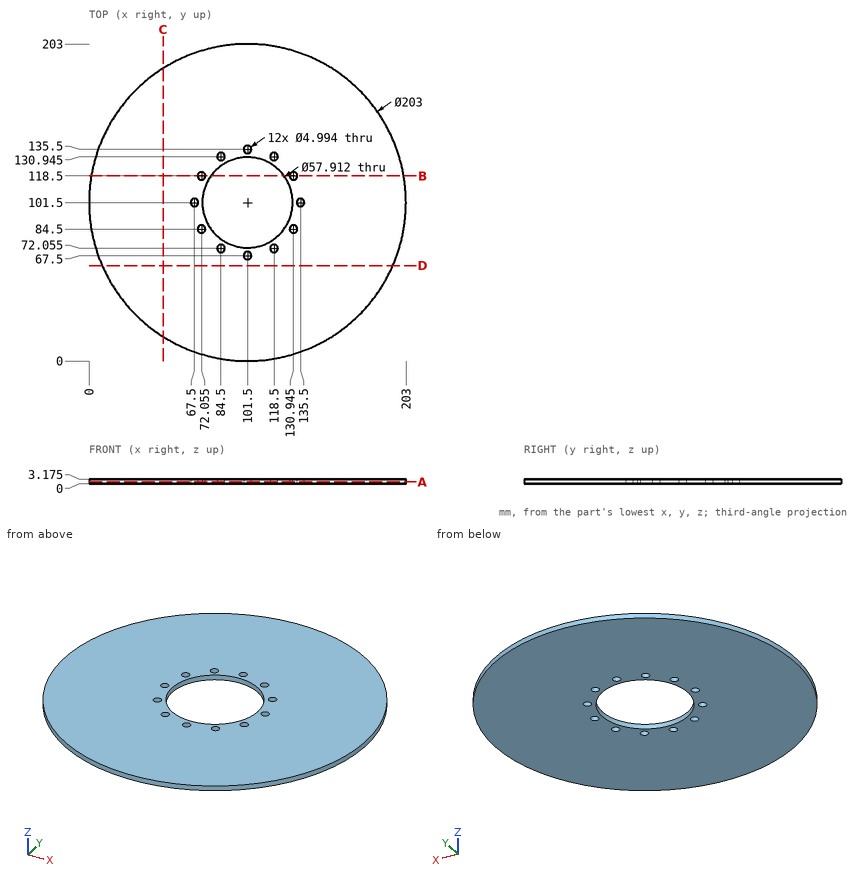
Answer from the drawing. Dimensions are ordinates in mm from the lowest x, y and z of the part. Coordinates: 2 decimals unless noted, no trailing zeros. Order: outer loops, then holes, each group sorted by start corner. A loop starts at its lowest first (then second) coordinate and runs counter-clockwise, first axis right, second up. Notation, with made-up numbers: (49.5, 38.25) -> (78.5, 38.25) arc R32 ccw to (78.5, 72.25) -> close; hole circle Ø9 at (5, -14.75). An arc over 180 degrees is marked (long way). Answer as a JSON object with one key per item and string values.
1) A cutting plane is placed at C-C, the plane x = 47.5. Determine the outline of the cut face in (y, z) (1 decimal), plus the area to 3 significant figures.
Model answer:
{"outline": "(15.6, 0) -> (187.4, 0) -> (187.4, 3.2) -> (15.6, 3.2) -> close", "area": "546 mm²"}
2) A cutting plane is placed at A-A, the plane z = 1.35. State how many separate pieces and enclosed holes the cut face has, plus the area to 3 significant figures.
Model answer:
{"separate pieces": "1", "enclosed holes": "13", "area": "29,500 mm²"}
3) Consider line 1 along X through (y, z) = (102, 2.3); line 2 along Y through (x, z) = (101.5, 2); line 3 along Y through (x, z) = (85.5, 2.3). Determine where each line is inside the solid, lowest interval first. Write a range as from..to.
Model answer:
{"line 1": "x = 0..65.05, 69.95..72.55, 130.45..133.05, 137.95..203", "line 2": "y = 0..65, 70..72.54, 130.46..133, 138..203", "line 3": "y = 1.27..69.77, 74.34..77.37, 125.63..128.66, 133.23..201.73"}
4) A cutting plane is placed at B-B, the plane y = 118.5. Determine the outline of the cut face in (x, z) (1 decimal), plus the area to 3 significant figures.
Model answer:
{"outline": "(1.4, 0) -> (69.6, 0) -> (69.6, 3.2) -> (1.4, 3.2) -> close; (74.6, 0) -> (78.1, 0) -> (78.1, 3.2) -> (74.6, 3.2) -> close; (124.9, 0) -> (128.4, 0) -> (128.4, 3.2) -> (124.9, 3.2) -> close; (133.4, 0) -> (201.6, 0) -> (201.6, 3.2) -> (133.4, 3.2) -> close", "area": "455 mm²"}
5) Each of these flat-tipped pins is pushed along its axis until it touches: pin 1 (4 mm diameter, centred on x = 67.5, y = 101.5, fed in from +Z); pin 2 (1.5 mm diameter, centred on x = 74.5, z = 1.5, fed in from -Y). Where does it stop, or does it pass through?
Model answer:
{"pin 1": "passes through", "pin 2": "stops at y = 3.45"}
6) A cutting plane is placed at D-D, the plane y = 61. Determine the outline of the cut face in (x, z) (3 decimals).
Model answer:
{"outline": "(8.43, 0) -> (194.57, 0) -> (194.57, 3.175) -> (8.43, 3.175) -> close"}
